The model under review builds one solid part; all positions refer to its coordinate system, in mm. Coordinates: 2 decimals unless noted, no trailing zeros. Write each loop counter-clockwise with the first axis right and the second up, starting at its lowest first coordinate (ties: lowest second). Pieces come first, ordered by that corner, then holes. Notation, with made-up numbers: M 53.5,69.5 L 74.5,69.5 A11 ccw 74.5,74.5 Z; hole C 61,5 d7. An arc over 180 degrees is marked long. Answer as CSV lines item,"result". Start each with the question number.
from build123d import *

# Parameters (mm, degrees)
CROQUIS1_W              = 63.5
CROQUIS1_H              = 12.5
SALIENTE_EXTRUIR1_DEPTH = 127
CORTAR_EXTRUIR1_DEPTH   = 127
REDONDEO1_R             = 10


with BuildPart() as part:
    # Croquis1 → Saliente-Extruir1 (new body)
    with BuildSketch(Plane.XY):
        Rectangle(CROQUIS1_W, CROQUIS1_H)
    extrude(amount=SALIENTE_EXTRUIR1_DEPTH)

    # Croquis2 → Cortar-Extruir1 (cut)
    with BuildSketch(Plane(origin=(0, 6.25, 0), x_dir=(1, 0, 0), z_dir=(0, 1, 0))):
        with BuildLine():
            ThreePointArc((0, -127), (-16.200333365, -125.368441446), (-31.75, -120.539295353))
            Line((-31.75, -120.539295353), (-31.75, -127))
            Line((-31.75, -127), (0, -127))
        make_face()
        with BuildLine():
            ThreePointArc((31.75, -120.539295353), (16.200333365, -125.368441446), (0, -127))
            Line((0, -127), (31.75, -127))
            Line((31.75, -127), (31.75, -120.539295353))
        make_face()
    extrude(amount=-CORTAR_EXTRUIR1_DEPTH, mode=Mode.SUBTRACT)

    # Redondeo1
    redondeo1_edges = [part.edges().sort_by_distance(p)[0] for p in [
        (-31.75, 0, 120.539295353),
        (31.75, 0, 120.539295353),
        (-31.75, 0, 0),
        (31.75, 0, 0),
    ]]
    fillet(redondeo1_edges, radius=REDONDEO1_R)


solid = part.part
1) To check wall thickness, follow line 1 (Z direction, x = 25, y = -4); line 2 (Z direction, x = -12.5, y = 1); line 3 (X direction, y = 2.75, z = 114.5). State the ranges of each line that lie inside material, in increasing order. Write a range as [from, to].
2) Clearance check with a flat-ended pin moving along its axis: pin 1 Ø3 at (x, y) = (20.5, 3.5) entering from +Z. State where the tip first meets the part, or that it passes through.
3) Take a section at B-B on x = 20. Give the boundary of the cut face in (y, z).
4) Take a section at C-C on x = 26.5. Give the boundary of the cut face in (y, z), and give its area (3 significant figures).
5) Take a section at A-A on y = -0.25. Give the boundary of the cut face in (x, z).
Results:
1,line 1,"z = [0.54, 123.06]"
1,line 2,"z = [0, 126.03]"
1,line 3,"x = [-31.71, 31.71]"
2,pin 1,"stops at z = 124.75"
3,outline,"M -6.25,0 L 6.25,0 L 6.25,124.5 L -6.25,124.5 Z"
4,outline,"M -6.25,1.2 L 6.25,1.2 L 6.25,122.4 L -6.25,122.4 Z"
4,area,"1,510 mm²"
5,outline,"M -31.75,10 A10 ccw -21.75,0 L 21.75,0 A10 ccw 31.75,10 L 31.75,113.6 A10 ccw 24.8,123.12 A81.25 ccw -24.8,123.12 A10 ccw -31.75,113.6 Z"
